from build123d import *

# Parameters (mm, degrees)
CROQUIS5_W            = 12
CROQUIS5_H            = 0.6
CORTAR_EXTRUIR2_DEPTH = 3


with BuildPart() as part:
    # Croquis2 → Revolución1 (revolve)
    with BuildSketch(Plane(origin=(0, 0, 7), x_dir=(0, 0, 1), z_dir=(-1, 0, 0)), mode=Mode.PRIVATE) as revoluci_n1_sk:
        Polygon((-7, 0), (-30, 0), (-30, 3), (-14.5, 3), (-14.5, 5.711324865), (-14, 6), (-7, 6), align=None)
    revolve(revoluci_n1_sk.sketch.rotate(Axis((0, 0, 0), (0, 0, -1)), 180), axis=Axis((0, 0, 0), (0, 0, -1)))

    # Croquis5 → Cortar-Extruir2 (cut, symmetric)
    with BuildSketch(Plane(origin=(0, 0, 0), x_dir=(0, 0, -1), z_dir=(1, 0, 0))):
        with Locations((17, 2.7)):
            Rectangle(CROQUIS5_W, CROQUIS5_H)
    extrude(amount=CORTAR_EXTRUIR2_DEPTH, both=True, mode=Mode.SUBTRACT)


solid = part.part
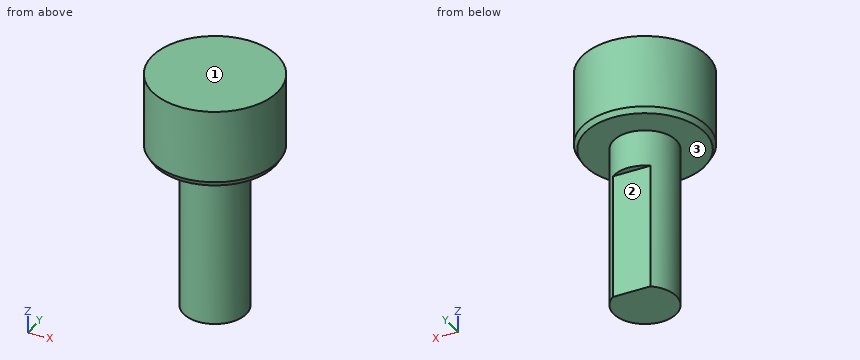
Work out the finished part from the listing and answer in its coordinate system (mm). Face numbers are marked on the shaded views. A direction names the side the tool comes from. Round coordinates to 2 decimals unless told otherwise and drop trailing zeros. Write each loop counter-clockwise with the first axis right and the second up, starting at its lowest first coordinate (ties: lowest second). Pieces come first, ordered by that corner, then holes. Notation, with made-up numbers: (-11, 40.5) -> (1, 40.5) arc R20 cw to (1, 57.5) -> close; hole circle Ø2 at (11.25, 40.5). An arc over 180 degrees is marked (long way). Write each question's results on one line, items separated by ' | '.
Item 1: A cutting plane is placed at A-A, the plane y = 0. Determine the outline of the cut face in (x, z), plus the area to 3 significant figures.
Result set:
outline: (-6, -7) -> (-5.71, -7.5) -> (-3, -7.5) -> (-3, -23) -> (3, -23) -> (3, -7.5) -> (5.71, -7.5) -> (6, -7) -> (6, 0) -> (-6, 0) -> close | area: 183 mm^2
Item 2: A cutting plane is placed at B-B, the plane z = -8.75. Determine the outline of the cut face in (x, y).
Result set:
outline: circle Ø6 at (0, 0)
Item 3: Find the intervals of material crossed by line 1 along Z through (x, y) = (2, -4.75); line 2 along X through (y, z) = (-0.25, -4.75); line 3 along Y through (x, z) = (5.5, -1.75), in increasing order. Write a range as [from, to].
Result set:
line 1: [-7.5, 0] | line 2: [-5.99, 5.99] | line 3: [-2.4, 2.4]
Item 4: Flat-ended cylindrical pins translate along their axes: P1, Ø1.5, axis at x = -1, z = -19.5, coming from the -Y side; P2, Ø3, axis at x = -0.5, z = -15, coming from the +Y side; P3, Ø1, axis at x = 4.5, z = -3.5, coming from the +Y side. Find the tip coordinate at first contact, or state that the pin passes through.
Result set:
P1: y = -2.99 | P2: y = 2.4 | P3: y = 4.47
Item 5: Which of the six approach directions +Z, -Z, +X, -X, +Y, -Y give full straight-line access (tool end or side, diameter ignored) to the marked faces 1, 2 and 3?
Result set:
face 1: +Z, +X, -X, +Y, -Y | face 2: -Z, +X, -X, +Y | face 3: -Z
Item 6: A cutting plane is placed at C-C, the plane z = -13.75. Determine the outline of the cut face in (x, y).
Result set:
outline: (-1.8, 2.4) arc R3 ccw (long way) to (1.8, 2.4) -> close
